For this review, take the finished solid that the model builds, in its own axes (mm). Face numbers are marked on the shaded views. A direction names the side the tool comes from. Coordinates: 2 decimals unless noted, no trailing zeros. Write each loop counter-clockwise with the first axis right and the second up, starting at its lowest first coordinate (ties: lowest second). Pieces come first, ordered by that corner, then holes.
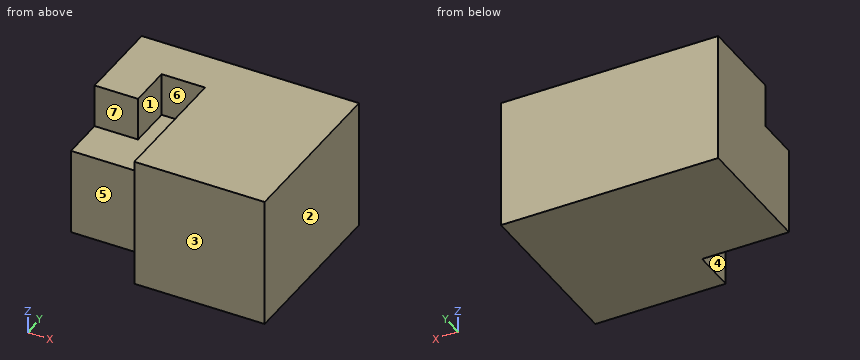
```python
from build123d import *

# Parameters (mm, degrees)
F0_W     = 25.4
F0_H     = 25.4
F1_DEPTH = 25.4
F2_DEPTH = 50.8
F3_DEPTH = 76.2
F4_DEPTH = 101.6


with BuildPart() as f1:
    # F0 (on Front) → F1 (new body)
    with BuildSketch(Plane.XZ):
        with Locations((-88.9, 63.5)):
            Rectangle(F0_W, F0_H)
    extrude(amount=F1_DEPTH)

    # F0 (on Front) → F2 (join)
    with BuildSketch(Plane.XZ):
        with Locations((-114.3, 63.5)):
            Rectangle(F0_W, F0_H)
    extrude(amount=F2_DEPTH)

    # F0 (on Front) → F3 (join)
    with BuildSketch(Plane.XZ):
        Polygon((-101.6, 50.8), (-127, 50.8), (-127, 0), (-76.2, 0), (-76.2, 50.8), align=None)
    extrude(amount=F3_DEPTH)

    # F0 (on Front) → F4 (join)
    with BuildSketch(Plane.XZ):
        Polygon((0, 76.2), (-76.2, 76.2), (-76.2, 50.8), (-76.2, 0), (0, 0), align=None)
    extrude(amount=F4_DEPTH)


solid = f1.part
```
Q1. Add section A-A (z = 70.5). State the section outline as (x, y) points, then the cut area to 3 significant figures.
Ans:
outline: (-127, -50.8) - (-101.6, -50.8) - (-101.6, -25.4) - (-76.2, -25.4) - (-76.2, -101.6) - (0, -101.6) - (0, 0) - (-127, 0) - close
area: 9,680 mm2
Q2. Tool access review of the marked faces 5, 6 and 7: name each direction out of +Z, -Z, +X, -X, +Y, -Y from which nothing blocks a thin tool from reaching the whole face with its end or side.
Ans:
face 5: +Z, -Z, -X, -Y
face 6: +Z, -Y
face 7: +Z, -X, -Y
Q3. Clearance check with flat-ended pins moving along their axes: pin 1 Ø7.5 at (x, z) = (-114.5, 59.5) entering from -Y; pin 2 Ø7.5 at (x, z) = (-90.5, 60) entering from -Y. State where each tip first meets the part, or that it passes through.
Ans:
pin 1: stops at y = -50.8
pin 2: stops at y = -25.4
Q4. Add section D-D (y = -81.5). State the section outline as (x, z) points.
Ans:
outline: (-76.2, 0) - (0, 0) - (0, 76.2) - (-76.2, 76.2) - close
Q5. Add section B-B (y = -56). State the section outline as (x, z) points.
Ans:
outline: (-127, 0) - (0, 0) - (0, 76.2) - (-76.2, 76.2) - (-76.2, 50.8) - (-127, 50.8) - close
Q6. Add section C-C (x = -104). State the section outline as (y, z) points, then the cut area to 3 significant figures.
Ans:
outline: (-76.2, 0) - (0, 0) - (0, 76.2) - (-50.8, 76.2) - (-50.8, 50.8) - (-76.2, 50.8) - close
area: 5,160 mm2
Q7. Draft analysis for pull direction X (two halves, no side actions). For the marked faces 1, 2, 3 and 4, state which applies: +X half, -X half, draft (parallel to the pull), parting line (faces both ways), or undercut.
Ans:
face 1: undercut
face 2: +X half
face 3: draft
face 4: undercut
Q8. For probe 1 along Y at (x, z) = (-96.5, 36); probe 2 along Z at (x, y) = (-85, -64.5), list the stretches that pass through material, from the lowest coordinate up.
Ans:
probe 1: y = -76.2 to 0
probe 2: z = 0 to 50.8
